Read the model definition and answer for the solid it produces. Units are mm, in the model's axes. A direction names the side the tool comes from. Give positions to 0.01 mm unless a question says otherwise; leave off trailing zeros. Write each loop counter-clockwise with the first axis right and the second up, starting at its lowest first coordinate (ties: lowest second). Pieces come first, ordered by that corner, then holes. Notation, with made-up numbers: (16.5, 19) -> (34.5, 19) arc R11 ccw to (34.5, 35) -> close; hole circle Ø3 at (-18.75, -11.75). An arc over 180 degrees is marked (long way). Answer as CSV lines item,"result". Start each with the question number.
1. The part is cut by section C-C, the plane z = 1.1. Determine the outline of the cut face in (x, y), and give its area (3 significant figures).
2. For a pull along Y with two mould halves and no side action, classify faces 1 (the cylindrical face through (39.97, -1.57, 1.78)), 2 (the flat face through (9, 9, 0)), 3 (the flat face through (-21, -8, 2)) as pulls with the +Y half, pulls with the -Y half, needs draft (parallel to the pull), parting line crosses it, or undercut.
3. The part is cut by section A-A, the plane x = 0. Determine the outline of the cut face in (y, z), and give its area (3 significant figures).
4. A tool of negligible diameter and unlimited length cuts with its end or side. For faces 4 (the flat face through (9, -8, 3)), 5 (the flat face through (-21, 8, 2)), from which of +Z, -Z, +X, -X, +Y, -Y can it reach the whole face along a straight path? Write none if from no direction.
5. Given pin 1 (0.7 mm diameter, centred on x = -15.5, z = 2.5, fed in from -Y); pin 2 (1.5 mm diameter, centred on y = 24.5, z = 0.5, fed in from +X); pin 3 (1.2 mm diameter, centred on x = -26.5, z = 2.5, fed in from +Y), each flat-ended and moving along its own axis, determine where each tip first touches the part or whether it passes through.
6. Find the intervals of material crossed by line 1 (Y direction, x = 0, z = 1.3); line 2 (Y direction, x = -20, z = 1.1); line 3 (X direction, y = -25.5, z = 0.75), in increasing order.
7. The part is cut by section B-B, the plane y = 0. Determine the outline of the cut face in (x, z), and give its area (3 significant figures).
from build123d import *

# Parameters (mm, degrees)
PAD_DEPTH    = 3
CHAMFER_SIZE = 0.6


with BuildPart() as part:
    # Sketch → Pad (new body)
    with BuildSketch(Plane.XY):
        with BuildLine():
            ThreePointArc((-37.712362, -13.333333), (40, 0), (-37.712362, 13.333333))
            ThreePointArc((-37.712362, 13.333333), (-37.207112, 9.690599), (-33.941125, 8))
            Line((-33.941125, 8), (-6.800735, 8))
            ThreePointArc((-6.800735, -8), (10.5, 0), (-6.800735, 8))
            Line((-33.941125, -8), (-6.800735, -8))
            ThreePointArc((-33.941125, -8), (-37.207112, -9.690599), (-37.712362, -13.333333))
        make_face()
    extrude(amount=PAD_DEPTH)

    # Chamfer
    chamfer_edges = [part.edges().sort_by_distance(p)[0] for p in [
        (-37.207112, -9.690599, 0),
        (40, 0, 0),
        (-37.207112, 9.690599, 0),
        (-20.37093, 8, 0),
        (10.5, 0, 0),
        (-20.37093, -8, 0),
    ]]
    chamfer(chamfer_edges, length=CHAMFER_SIZE)


solid = part.part
Results found:
1,outline,"(-37.71, -13.33) arc R40 ccw (long way) to (-37.71, 13.33) arc R4 ccw to (-33.94, 8) -> (-6.8, 8) arc R10.5 cw (long way) to (-6.8, -8) -> (-33.94, -8) arc R4 ccw to start"
1,area,"4,180 mm²"
2,face 1,"parting line crosses it"
2,face 2,"needs draft"
2,face 3,"undercut"
3,outline,"(-40, 0.6) -> (-39.4, 0) -> (-11.1, 0) -> (-10.5, 0.6) -> (-10.5, 3) -> (-40, 3) -> close; (10.5, 0.6) -> (11.1, 0) -> (39.4, 0) -> (40, 0.6) -> (40, 3) -> (10.5, 3) -> close"
3,area,"176 mm²"
4,face 4,"+Z, +X, -X, +Y, -Y"
4,face 5,"+Z, -Z, -X"
5,pin 1,"stops at y = -37.02"
5,pin 2,"stops at x = 32.18"
5,pin 3,"stops at y = 30.48"
6,line 1,"y = -40 to -10.5, 10.5 to 40"
6,line 2,"y = -34.64 to -8, 8 to 34.64"
6,line 3,"x = -30.82 to 30.82"
7,outline,"(10.5, 0.6) -> (11.1, 0) -> (39.4, 0) -> (40, 0.6) -> (40, 3) -> (10.5, 3) -> close"
7,area,"88.1 mm²"
